Work out the finished part from the listing and answer in its coordinate system (mm). Face numbers are marked on the shaded views. A direction names the side the tool comes from. Give positions to 0.01 mm unless a question says otherwise; leave off trailing zeros. Loops run counter-clockwise (first coordinate to the right, second up) from the corner with the lowest first, then second, coordinate; pieces in that order, holes last.
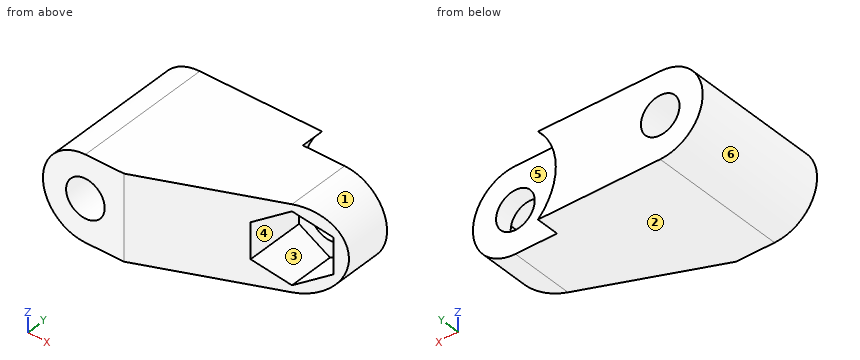
```python
from build123d import *

# Parameters (mm, degrees)
CROQUIS1_R                 = 2.5
SALIENTE_EXTRUIR1_DEPTH    = 15
CORTAR_EXTRUIR1_DEPTH      = 15
CORTAR_EXTRUIR2_DEPTH      = 3.7
CORTAR_EXTRUIR2_DEPTH_BACK = 15
CROQUIS4_R                 = 2.5
SALIENTE_EXTRUIR2_DEPTH    = 3


with BuildPart() as part:
    # Croquis1 → Saliente-Extruir1 (new body)
    with BuildSketch(Plane(origin=(0, 0, 0), x_dir=(1, 0, 0), z_dir=(0, 1, 0))):
        with BuildLine():
            Line((0, 5.5), (21.215, 5.5))
            ThreePointArc((21.215, 5.5), (26.715, 0), (21.215, -5.5))
            Line((21.215, -5.5), (0, -5.5))
            ThreePointArc((0, -5.5), (-5.5, 0), (0, 5.5))
        make_face()
        with Locations(Location((0, 0, 0), (0, 0, 270))):
            Circle(CROQUIS1_R, mode=Mode.SUBTRACT)
        with Locations(Location((21.215, 0, 0), (0, 0, 270))):
            Circle(CROQUIS1_R, mode=Mode.SUBTRACT)
    extrude(amount=SALIENTE_EXTRUIR1_DEPTH)

    # Croquis2 → Cortar-Extruir1 (cut)
    with BuildSketch(Plane.XY.offset(5.5)):
        Polygon((5, 0), (26.715, 9), (26.715, 0), align=None)
    extrude(amount=-CORTAR_EXTRUIR1_DEPTH, mode=Mode.SUBTRACT)

    # Croquis3 → Cortar-Extruir2 (cut, two sides: drawn at the far end of the back side and taken through both)
    with BuildSketch(Plane(origin=(0, 9, 0), x_dir=(1, 0, 0), z_dir=(0, 1, 0)).offset(-CORTAR_EXTRUIR2_DEPTH_BACK)):
        Polygon((17.215, 2.309401077), (17.215, -2.309401077), (21.215, -4.618802154), (25.215, -2.309401077), (25.215, 2.309401077), (21.215, 4.618802154), align=None)
    extrude(amount=CORTAR_EXTRUIR2_DEPTH + CORTAR_EXTRUIR2_DEPTH_BACK, mode=Mode.SUBTRACT)

    # Croquis4 → Saliente-Extruir2 (add)
    with BuildSketch(Plane(origin=(0, 15, 0), x_dir=(1, 0, 0), z_dir=(0, 1, 0))):
        with BuildLine():
            Line((0, -5.5), (15.826122566, -5.5))
            ThreePointArc((15.826122566, -5.5), (13.515, 0), (15.826122566, 5.5))
            Line((15.826122566, 5.5), (0, 5.5))
            ThreePointArc((0, 5.5), (-5.5, 0), (0, -5.5))
        make_face()
        with Locations(Location((0, 0, 0), (0, 0, 270))):
            Circle(CROQUIS4_R, mode=Mode.SUBTRACT)
    extrude(amount=SALIENTE_EXTRUIR2_DEPTH)


solid = part.part
```
Q1. Consider line 1 along X through (y, z) = (13.8, 0) (3 decimals); line 2 along X through (y, z) = (7.5, 0) (3 decimals); line 3 along Z through (x, y) = (-2, 9.5). Determine where each line is inside the solid, lowest interval first.
Q2. Section C-C on z = 0 is taken. Give the vertices of the cut face in (x, y) (3 decimals).
Q3. Section A-A on x = 0.5 is taken. Give the vertices of the cut face in (y, z).
Q4. Which of the six approach directions +Z, -Z, +X, -X, +Y, -Y give full straight-line access (tool end or side, diameter ignored) to the marked faces 4, 5 and 6?
Q5. Section D-D on x = 23 is taken. Give the vertices of the cut face in (y, z), plus the area to 3 significant figures.
Q6. Given pin 1 (1.5 mm diameter, centred on x = -1.5, y = 4, fed in from -Z); pin 2 (6 mm diameter, centred on x = 23, y = 10, fed in from +Z); pin 3 (4 mm diameter, centred on x = 0, z = 0, fed in from +Y); pin 4 (6 mm diameter, centred on x = 21.215, z = 0, fed in from +Y), each flat-ended and moving along its own axis, determine where each tip first touches the part or whether it passes through.
Q7. Section B-B on y = 10 is taken. Give the vertices of the cut face in (x, z) (3 decimals), plus the area to 3 significant figures.
Q8. Determine the mould class of the marked faces 1, 2 and 3 for opening direction Z: +Z half, -Z half, draft (parallel to the pull), parting line (faces both ways), or undercut.
Check result:
1. line 1: x = -5.5 to -2.5, 2.5 to 18.715, 23.715 to 26.715
1. line 2: x = -5.5 to -2.5, 2.5 to 17.215
1. line 3: z = -5.12 to -1.5, 1.5 to 5.12
2. outline: (-5.5, 0) - (-2.5, 0) - (-2.5, 18) - (-5.5, 18) - close; (2.5, 0) - (5, 0) - (17.215, 5.063) - (17.215, 12.7) - (18.715, 12.7) - (18.715, 15) - (13.515, 15) - (13.515, 18) - (2.5, 18) - close; (23.715, 12.7) - (25.215, 12.7) - (25.215, 8.378) - (26.715, 9) - (26.715, 15) - (23.715, 15) - close
3. outline: (0, -5.5) - (18, -5.5) - (18, -2.45) - (0, -2.45) - close; (0, 2.45) - (18, 2.45) - (18, 5.5) - (0, 5.5) - close
4. face 4: -Y
4. face 5: +X, +Y
4. face 6: -X, +Y, -Y
5. outline: (7.46, -5.2) - (15, -5.2) - (15, -1.75) - (12.7, -1.75) - (12.7, -3.59) - (7.46, -3.59) - close; (7.46, 3.59) - (12.7, 3.59) - (12.7, 1.75) - (15, 1.75) - (15, 5.2) - (7.46, 5.2) - close
5. area: 32.8 mm2
6. pin 1: stops at z = -5.45
6. pin 2: stops at z = 5.5
6. pin 3: passes through
6. pin 4: stops at y = 15
7. outline: (0, -5.5) - (21.215, -5.5) arc R5.5 ccw to (21.215, 5.5) - (0, 5.5) arc R5.5 ccw to start; hole circle Ø5 at (0, 0); hole (17.215, -2.309) - (21.215, -4.619) - (25.215, -2.309) - (25.215, 2.309) - (21.215, 4.619) - (17.215, 2.309) - close
7. area: 253 mm2
8. face 1: parting line
8. face 2: -Z half
8. face 3: undercut
